Design review of the part built by this model. Coordinates are the model's own, in mm. Face numbers are marked on the shaded views. A direction names the side the tool comes from. Coordinates: 2 decimals unless noted, no trailing zeros. Write each loop counter-clockwise with the first axis right and the second up, starting at its lowest first coordinate (ties: lowest second). Pieces come first, ordered by that corner, then holes.
Q1. The part is to be moulded in two halves that separate along X. For the marked faces 4, 5 and 6, say which applies: +X half, -X half, draft (parallel to the pull), parting line (faces both ways), or undercut.
Q2. Machinability: for the marked faces 1, 2 and 3, which of the approach directions +Z, -Z, +X, -X, +Y, -Y give a long, thin tool a straight path to every point of the face, cutting with its end or side? Answer none if there is none.
Q3. Clearance check with flat-ended pins moving along their axes: pin 1 Ø15 at (y, z) = (31.5, 164) entering from +X; pin 2 Ø8 at (x, y) = (121, 21.5) entering from -Z; pin 3 Ø1.8 at (y, z) = (12, 15.5) entering from +X; pin 4 Ø5 at (x, z) = (71.5, -33) entering from -Y. State where each tip first meets the part, or that it passes through.
Q4. Add section A-A, the plane x = 0. Give the boundary of the cut face in (y, z), plus the area to 3 significant figures.
Q5. To check wall thickness, follow probe 1 along X at (y, z) = (33.5, -5); probe 2 along Y at (x, z) = (-1.5, -139.5); probe 3 along X at (y, z) = (64, -161). State the ranges of each line that lie inside material, in increasing order.
from build123d import *

# Parameters (mm, degrees)
SKETCH1_R                = 150
BOSS_EXTRUDE1_DEPTH      = 75
CHAMFER1_SIZE            = 10
BOSS_EXTRUDE2_START      = -75
BOSS_EXTRUDE2_DEPTH      = 10
CHAMFER2_SIZE            = 7
BOSS_EXTRUDE3_DEPTH      = 9
BOSS_EXTRUDE4_DEPTH      = 3.5
CIRPATTERN1_COUNT        = 4
CIRPATTERN1_COPY_1_DEPTH = 9
CIRPATTERN1_COPY_2_DEPTH = 9
CIRPATTERN1_COPY_3_DEPTH = 9
CIRPATTERN1_COPY_4_DEPTH = 3.5
CIRPATTERN1_COPY_5_DEPTH = 3.5
CIRPATTERN1_COPY_6_DEPTH = 3.5
CUT_EXTRUDE1_START       = -60
CUT_EXTRUDE1_DEPTH       = 60
SKETCH6_R                = 110
BOSS_EXTRUDE5_DEPTH      = 9
BOSS_EXTRUDE5_TAPER      = 45
SKETCH7_R                = 15
BOSS_EXTRUDE6_DEPTH      = 20


with BuildPart() as part:
    # Sketch1 → Boss-Extrude1 (new body)
    with BuildSketch(Plane(origin=(0, 0, 0), x_dir=(1, 0, 0), z_dir=(0, 1, 0))):
        with Locations(Location((0, 0, 0), (0, 0, 270))):
            Circle(SKETCH1_R)
    extrude(amount=BOSS_EXTRUDE1_DEPTH)

    # Chamfer1
    chamfer1_edges = [part.edges().sort_by_distance(p)[0] for p in [
        (0, 75, -150),
    ]]
    chamfer(chamfer1_edges, length=CHAMFER1_SIZE)

    # Sketch2 → Boss-Extrude2 (add)
    with BuildSketch(Plane(origin=(0, 75, 0), x_dir=(1, 0, 0), z_dir=(0, 1, 0)).offset(BOSS_EXTRUDE2_START)):
        with BuildLine():
            Line((-145.236875483, 37.5), (-195.236875483, 37.5))
            Line((-195.236875483, 37.5), (-195.236875483, -37.5))
            Line((-195.236875483, -37.5), (-145.236875483, -37.5))
            ThreePointArc((-145.236875483, -37.5), (-150, 0), (-145.236875483, 37.5))
        make_face()
    boss_extrude2 = extrude(amount=BOSS_EXTRUDE2_DEPTH)

    # Chamfer2
    chamfer2_edges = [part.edges().sort_by_distance(p)[0] for p in [
        (-195.236875483, 5, -37.5),
        (-195.236875483, 5, 37.5),
    ]]
    chamfer(chamfer2_edges, length=CHAMFER2_SIZE)

    # Sketch3 → Boss-Extrude3 (add)
    with BuildSketch(Plane.XY.offset(37.5)):
        Polygon((-145.236875483, 10), (-145.236875483, 65), (-170.556875483, 65), (-188.236875483, 10), align=None)
    boss_extrude3 = extrude(amount=-BOSS_EXTRUDE3_DEPTH)

    # Sketch4 → Boss-Extrude4 (add)
    with BuildSketch(Plane(origin=(0, 10, 0), x_dir=(1, 0, 0), z_dir=(0, 1, 0))):
        Polygon((-183.04072306, -12), (-188.236875483, -9), (-193.433027905, -12), (-193.433027905, -18), (-188.236875483, -21), (-183.04072306, -18), align=None)
    boss_extrude4 = extrude(amount=BOSS_EXTRUDE4_DEPTH)

    # Mirror1: Boss-Extrude3, Boss-Extrude4 across plane
    add(boss_extrude3.mirror(Plane.XY))
    add(boss_extrude4.mirror(Plane.XY))

    # CirPattern1: Boss-Extrude2, Boss-Extrude3, Boss-Extrude4 ×4 about axis
    cirpattern1_axis = Axis((0, 0, 0), (0, 1, 0))
    add([boss_extrude2.rotate(cirpattern1_axis, i * 360 / CIRPATTERN1_COUNT) for i in range(1, CIRPATTERN1_COUNT)])
    add([boss_extrude3.rotate(cirpattern1_axis, i * 360 / CIRPATTERN1_COUNT) for i in range(1, CIRPATTERN1_COUNT)])
    add([boss_extrude4.rotate(cirpattern1_axis, i * 360 / CIRPATTERN1_COUNT) for i in range(1, CIRPATTERN1_COUNT)])

    # CirPattern1 copy 1 sketch → CirPattern1 copy 1 (add)
    with BuildSketch(Plane(origin=(-37.5, 0, 0), x_dir=(0, 0, -1), z_dir=(-1, 0, 0))):
        Polygon((-145.236875483, -10), (-145.236875483, -65), (-170.556875483, -65), (-188.236875483, -10), align=None)
    extrude(amount=-CIRPATTERN1_COPY_1_DEPTH)

    # CirPattern1 copy 2 sketch → CirPattern1 copy 2 (add)
    with BuildSketch(Plane(origin=(0, 0, 37.5), x_dir=(-1, 0, 0), z_dir=(0, 0, 1))):
        Polygon((-145.236875483, -10), (-145.236875483, -65), (-170.556875483, -65), (-188.236875483, -10), align=None)
    extrude(amount=-CIRPATTERN1_COPY_2_DEPTH)

    # CirPattern1 copy 3 sketch → CirPattern1 copy 3 (add)
    with BuildSketch(Plane(origin=(37.5, 0, 0), x_dir=(0, 0, 1), z_dir=(1, 0, 0))):
        Polygon((-145.236875483, -10), (-145.236875483, -65), (-170.556875483, -65), (-188.236875483, -10), align=None)
    extrude(amount=-CIRPATTERN1_COPY_3_DEPTH)

    # CirPattern1 copy 4 sketch → CirPattern1 copy 4 (add)
    with BuildSketch(Plane(origin=(0, 10, 0), x_dir=(0, 0, -1), z_dir=(0, 1, 0))):
        Polygon((-183.04072306, 12), (-188.236875483, 9), (-193.433027905, 12), (-193.433027905, 18), (-188.236875483, 21), (-183.04072306, 18), align=None)
    extrude(amount=CIRPATTERN1_COPY_4_DEPTH)

    # CirPattern1 copy 5 sketch → CirPattern1 copy 5 (add)
    with BuildSketch(Plane(origin=(0, 10, 0), x_dir=(-1, 0, 0), z_dir=(0, 1, 0))):
        Polygon((-183.04072306, 12), (-188.236875483, 9), (-193.433027905, 12), (-193.433027905, 18), (-188.236875483, 21), (-183.04072306, 18), align=None)
    extrude(amount=CIRPATTERN1_COPY_5_DEPTH)

    # CirPattern1 copy 6 sketch → CirPattern1 copy 6 (add)
    with BuildSketch(Plane.ZX.offset(10)):
        Polygon((-183.04072306, 12), (-188.236875483, 9), (-193.433027905, 12), (-193.433027905, 18), (-188.236875483, 21), (-183.04072306, 18), align=None)
    extrude(amount=CIRPATTERN1_COPY_6_DEPTH)

    # Sketch5 → Cut-Extrude1 (cut)
    with BuildSketch(Plane(origin=(0, 75, 0), x_dir=(1, 0, 0), z_dir=(0, 1, 0)).offset(CUT_EXTRUDE1_START)):
        with BuildLine():
            ThreePointArc((-65, -112.583302492), (-91.923881554, -91.923881554), (-112.583302492, -65))
            Line((-112.583302492, -65), (-121.24355653, -70))
            ThreePointArc((-121.24355653, -70), (-98.994949366, -98.994949366), (-70, -121.24355653))
            Line((-70, -121.24355653), (-65, -112.583302492))
        make_face()
        with BuildLine():
            ThreePointArc((-70, -121.24355653), (-98.994949366, -98.994949366), (-121.24355653, -70))
            Line((-121.24355653, -70), (-129.903810568, -75))
            ThreePointArc((-129.903810568, -75), (-106.066017178, -106.066017178), (-75, -129.903810568))
            Line((-75, -129.903810568), (-70, -121.24355653))
        make_face()
    extrude(amount=CUT_EXTRUDE1_DEPTH, mode=Mode.SUBTRACT)

    # Sketch6 → Boss-Extrude5 (add)
    with BuildSketch(Plane(origin=(0, 75, 0), x_dir=(1, 0, 0), z_dir=(0, 1, 0))):
        Circle(SKETCH6_R)
    extrude(amount=BOSS_EXTRUDE5_DEPTH, taper=BOSS_EXTRUDE5_TAPER)

    # Sketch7 → Boss-Extrude6 (add)
    with BuildSketch(Plane(origin=(0, 84, 0), x_dir=(1, 0, 0), z_dir=(0, 1, 0))):
        with Locations(Location((0, 0, 0), (0, 0, 270))):
            Circle(SKETCH7_R)
    extrude(amount=BOSS_EXTRUDE6_DEPTH)


solid = part.part
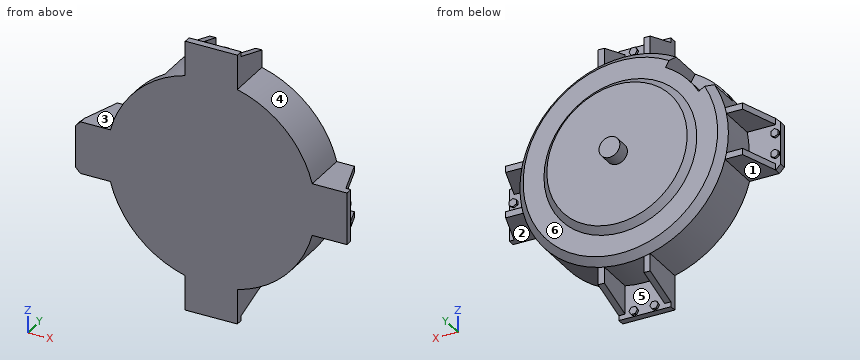
Here are the results:
1. face 4: +X half
1. face 5: undercut
1. face 6: draft
2. face 1: -Z, -X, +Y, -Y
2. face 2: -Z, +X, +Y, -Y
2. face 3: +Z, -X, +Y, -Y
3. pin 1: stops at x = 37.5
3. pin 2: stops at z = -93.87
3. pin 3: stops at x = 193.43
3. pin 4: stops at y = 0
4. outline: (0, -195.24) - (10, -195.24) - (10, -150) - (65, -150) - (75, -140) - (75, -110) - (84, -101) - (84, -15) - (104, -15) - (104, 15) - (84, 15) - (84, 101) - (75, 110) - (75, 140) - (65, 150) - (10, 150) - (10, 195.24) - (0, 195.24) - close
4. area: 25,800 mm2
5. probe 1: x = -149.92 to 149.92
5. probe 2: y = 0 to 75
5. probe 3: x = -37.5 to -28.5, 28.5 to 37.5
